```python
from build123d import *

# Parameters (mm, degrees)
EXTRUDE_1_DEPTH     = 13
SKETCH_2_R          = 2.5
CUT_EXTRUDE_1_DEPTH = 13
SKETCH_3_R          = 2.4
CUT_EXTRUDE_2_DEPTH = 13


with BuildPart() as part:
    # 草图1 → 凸台-拉伸1 (new body)
    with BuildSketch(Plane.XY):
        with BuildLine():
            Line((-12, -9.7), (-26.5, -9.7))
            Line((-26.5, -9.7), (-26.5, -15))
            Line((-26.5, -15), (26.5, -15))
            Line((26.5, -15), (26.5, -9.7))
            Line((26.5, -9.7), (12, -9.7))
            Line((12, -9.7), (12, 0))
            ThreePointArc((12, 0), (0, 12), (-12, 0))
            Line((-12, 0), (-12, -9.7))
        make_face()
    extrude(amount=EXTRUDE_1_DEPTH)

    # 草图2 → 切除-拉伸1 (cut)
    with BuildSketch(Plane.XY.offset(13)):
        Circle(SKETCH_2_R)
    extrude(amount=-CUT_EXTRUDE_1_DEPTH, mode=Mode.SUBTRACT)

    # 草图3 → 切除-拉伸2 (cut)
    with BuildSketch(Plane(origin=(0, -9.7, 0), x_dir=(1, 0, 0), z_dir=(0, 1, 0))):
        with Locations(Location((20, -6.5, 0), (0, 0, 180))):
            Circle(SKETCH_3_R)
        with Locations(Location((-20, -6.5, 0), (0, 0, 180))):
            Circle(SKETCH_3_R)
    extrude(amount=-CUT_EXTRUDE_2_DEPTH, mode=Mode.SUBTRACT)


solid = part.part
```
Check sheet for the modelled part. Datum: model origin and axes. Units: mm. A direction names the side the tool comes from. Give positions to 0.01 mm unless a question says otherwise; leave off trailing zeros. Order: outer loops, then holes, each group sorted by start corner. A loop starts at its lowest first (then second) coordinate and runs counter-clockwise, first axis right, second up. Notation, with made-up numbers: M 62.5,36 L 99.5,36 A22 ccw 99.5,58 Z; hole C 69.25,49.25 d11. An arc over 180 degrees is marked long. Answer in a Markdown table with one row per item.
1) Thickness scan on L1, parallel to Y at x = 0, z = 3.25; L2, parallel to Z at x = 20, y = -13.4; L3, parallel to X at y = -3.25, z = 8.75. Record the ranges inside material, lowest first. Write a range as [from, to].
Filled sheet:
| item | result |
|---|---|
| L1 | y = [-15, -2.5], [2.5, 12] |
| L2 | z = [0, 4.1], [8.9, 13] |
| L3 | x = [-12, 12] |
2) Gauge pin test, flat ends, axial feed: P1, Ø5, axis at y = -5.5, z = 5.5, coming from the -X side; P2, Ø4, axis at x = -16.5, z = 7, coming from the +Y side; P3, Ø3, axis at y = -5, z = 4.5, coming from the +X side. Record the tip position at first contact, or that the pin passes through.
Filled sheet:
| item | result |
|---|---|
| P1 | stops at x = -12 |
| P2 | stops at y = -9.7 |
| P3 | stops at x = 12 |
3) Cross-section at A-A, the plane z = 6.5. Enter the section's corners in (x, y).
Filled sheet:
| item | result |
|---|---|
| outline | M -26.5,-15 L -22.4,-15 L -22.4,-9.7 L -26.5,-9.7 Z; M -17.6,-15 L 17.6,-15 L 17.6,-9.7 L 12,-9.7 L 12,0 A12 ccw -12,0 L -12,-9.7 L -17.6,-9.7 Z; M 22.4,-15 L 26.5,-15 L 26.5,-9.7 L 22.4,-9.7 Z; hole C 0,0 d5 |
4) Cross-section at D-D, the plane x = 0. Enter the section's corners in (y, z), plus the area to 3 significant figures.
Filled sheet:
| item | result |
|---|---|
| outline | M -15,0 L -2.5,0 L -2.5,13 L -15,13 Z; M 2.5,0 L 12,0 L 12,13 L 2.5,13 Z |
| area | 286 mm2 |
5) Access from +Z, -Z, +X, -X, +Y, -Y to the whole of each face (thin tool, end or side, straight path). Record for faces 1 (the flat face through (-26.5, -12, 6)), 2 (the flat face through (17.7, -9.7, 5)), 3 (the flat face through (-12, -5, 6)).
Filled sheet:
| item | result |
|---|---|
| face 1 | +Z, -Z, -X, +Y, -Y |
| face 2 | +Z, -Z, +X, +Y |
| face 3 | +Z, -Z, -X, +Y |
6) Cross-section at B-B, the plane x = 20. Enter the section's corners in (y, z).
Filled sheet:
| item | result |
|---|---|
| outline | M -15,0 L -9.7,0 L -9.7,4.1 L -15,4.1 Z; M -15,8.9 L -9.7,8.9 L -9.7,13 L -15,13 Z |
7) Release check for a two-part mould opening along X. For faces 4 (the flat face through (26.5, -12, 6)), 5 (the cylindrical face through (0, 12, 6)), 6 (the cylindrical face through (22.398, -12.313, 6.606)), 7 (the cylindrical face through (-17.602, -12.313, 6.606)) record: +X half, -X half, draft (parallel to the pull), parting line (faces both ways), or undercut.
Filled sheet:
| item | result |
|---|---|
| face 4 | +X half |
| face 5 | parting line |
| face 6 | undercut |
| face 7 | undercut |
8) Cross-section at C-C, the plane z = 10.5. Enter the section's corners in (x, y).
Filled sheet:
| item | result |
|---|---|
| outline | M -26.5,-15 L 26.5,-15 L 26.5,-9.7 L 12,-9.7 L 12,0 A12 ccw -12,0 L -12,-9.7 L -26.5,-9.7 Z; hole C 0,0 d5 |
